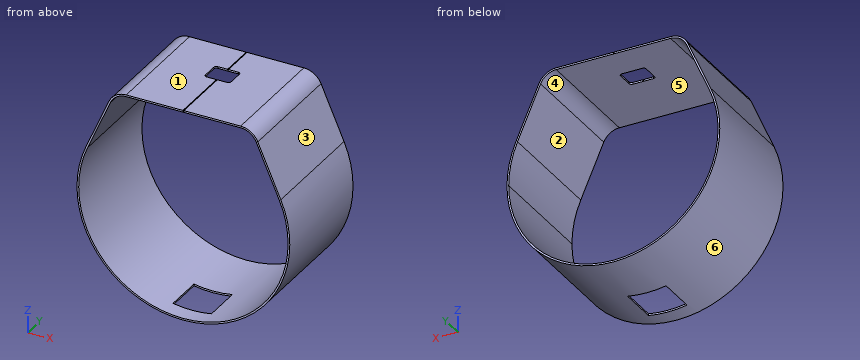
```python
from build123d import *

# Parameters (mm, degrees)
BOSS_EXTRUDE1_DEPTH = 90
CUT_EXTRUDE1_DEPTH  = 22
SKETCH4_W           = 22.5
SKETCH4_H           = 22.5
CUT_EXTRUDE3_DEPTH  = 126.897279558
CUT_EXTRUDE4_DEPTH  = 3
SKETCH6_W           = 0.5
SKETCH6_H           = 68
CUT_EXTRUDE5_DEPTH  = 0.5


# Read off the part's stored shape, not the designer's step: Cut-Extrude1
with BuildPart() as part:
    # Sketch1 → Boss-Extrude1 (new body)
    with BuildSketch(Plane(origin=(0, 0, 0), x_dir=(1, 0, 0), z_dir=(0, 1, 0))):
        with BuildLine():
            ThreePointArc((33.469387755, -62.25), (39.484065665, -60.45997555), (43.541212573, -55.672481752))
            Line((43.541212573, -55.672481752), (56.997372263, -25.027226277))
            ThreePointArc((56.997372263, -25.027226277), (0, 62.25), (-56.997372263, -25.027226277))
            Line((-56.997372263, -25.027226277), (-43.541212573, -55.672481752))
            ThreePointArc((-43.541212573, -55.672481752), (-39.484065665, -60.45997555), (-33.469387755, -62.25))
            Line((-33.469387755, -62.25), (33.469387755, -62.25))
        make_face()
        with BuildLine():
            Line((-9.5e-08, -61.25), (-33.469387755, -61.25))
            ThreePointArc((-33.469387755, -61.25), (-38.937276764, -59.622705046), (-42.625592135, -55.270437956))
            Line((-42.625592135, -55.270437956), (-56.081751825, -24.625182482))
            ThreePointArc((-56.081751825, -24.625182482), (-12.580842594, 59.944014711), (61.25, 0))
            ThreePointArc((61.25, 0), (59.944014711, -12.580842594), (56.081751825, -24.625182482))
            Line((56.081751825, -24.625182482), (42.625592135, -55.270437956))
            ThreePointArc((42.625592135, -55.270437956), (38.937276764, -59.622705046), (33.469387755, -61.25))
            Line((33.469387755, -61.25), (-9.5e-08, -61.25))
        make_face(mode=Mode.SUBTRACT)
    extrude(amount=BOSS_EXTRUDE1_DEPTH)

    # Cut-Extrude1 outline → Cut-Extrude1 (cut)
    with BuildSketch(Plane(origin=(0, 0, 0), x_dir=(1, 0, 0), z_dir=(0, 1, 0))):
        with BuildLine():
            Line((43.541212573, -55.672481752), (56.997372263, -25.027226277))
            ThreePointArc((56.997372263, -25.027226277), (0, 62.25), (-56.997372263, -25.027226277))
            Line((-56.997372263, -25.027226277), (-43.541212573, -55.672481752))
            ThreePointArc((-43.541212573, -55.672481752), (-39.484065665, -60.45997555), (-33.469387755, -62.25))
            Line((-33.469387755, -62.25), (33.469387755, -62.25))
            ThreePointArc((33.469387755, -62.25), (39.484065665, -60.45997555), (43.541212573, -55.672481752))
        make_face()
        with BuildLine():
            Line((33.469387755, -61.25), (-33.469387755, -61.25))
            ThreePointArc((-33.469387755, -61.25), (-38.937276765, -59.622705046), (-42.625592135, -55.270437956))
            Line((-42.625592135, -55.270437956), (-56.081751825, -24.625182482))
            ThreePointArc((-56.081751825, -24.625182482), (0, 61.25), (56.081751825, -24.625182482))
            Line((56.081751825, -24.625182482), (42.625592135, -55.270437956))
            ThreePointArc((42.625592135, -55.270437956), (38.937276765, -59.622705046), (33.469387755, -61.25))
        make_face(mode=Mode.SUBTRACT)
    extrude(amount=CUT_EXTRUDE1_DEPTH, mode=Mode.SUBTRACT)

    # Sketch4 → Cut-Extrude3 (cut, through all)
    with BuildSketch(Plane.XY):
        with Locations((0, 42.75)):
            Rectangle(SKETCH4_W, SKETCH4_H)
    extrude(amount=-CUT_EXTRUDE3_DEPTH, mode=Mode.SUBTRACT)

    # Sketch5 → Cut-Extrude4 (cut)
    with BuildSketch(Plane.XY.offset(62.25)):
        with BuildLine():
            Line((-6, 58), (6, 58))
            ThreePointArc((6, 58), (7.060660172, 58.439339828), (7.5, 59.5))
            Line((7.5, 59.5), (7.5, 68.5))
            ThreePointArc((7.5, 68.5), (7.060660172, 69.560660172), (6, 70))
            Line((6, 70), (-6, 70))
            ThreePointArc((-6, 70), (-7.060660172, 69.560660172), (-7.5, 68.5))
            Line((-7.5, 68.5), (-7.5, 59.5))
            ThreePointArc((-7.5, 59.5), (-7.060660172, 58.439339828), (-6, 58))
        make_face()
    extrude(amount=-CUT_EXTRUDE4_DEPTH, mode=Mode.SUBTRACT)

    # Sketch6 → Cut-Extrude5 (cut)
    with BuildSketch(Plane.XY.offset(62.25)):
        with Locations((0, 56)):
            Rectangle(SKETCH6_W, SKETCH6_H)
    extrude(amount=-CUT_EXTRUDE5_DEPTH, mode=Mode.SUBTRACT)


solid = part.part
```
Geometry check sheet. Reference: the model listing, model coordinates, mm. Face numbers are marked on the shaded views. A direction names the side the tool comes from. Give positions to 0.01 mm unless a question says otherwise; leave off trailing zeros. Write each loop counter-clockwise with the first axis right and the second up, starting at its lowest first coordinate (ties: lowest second). Pieces come first, ordered by that corner, then holes. Notation, with made-up numbers: (-19.5, 39.25) -> (27.5, 39.25) arc R28 cw to (27.5, 77.25) -> close; hole circle Ø3 at (-32.75, 41). An arc over 180 degrees is marked (long way). One line per question, with ' | ' between items.
Item 1: Sectioned sample at A-A, the plane y = 83. Record the boundary of the cut face in (x, z), plus the area to 3 significant figures.
Determined:
outline: (-57, 25.03) arc R62.25 ccw (long way) to (57, 25.03) -> (43.54, 55.67) arc R11 ccw to (33.47, 62.25) -> (0.25, 62.25) -> (0.25, 61.75) -> (-0.25, 61.75) -> (-0.25, 62.25) -> (-33.47, 62.25) arc R11 ccw to (-43.54, 55.67) -> close; hole (-56.08, 24.63) arc R61.25 ccw (long way) to (56.08, 24.63) -> (42.63, 55.27) arc R10 ccw to (33.47, 61.25) -> (-33.47, 61.25) arc R10 ccw to (-42.63, 55.27) -> close | area: 403 mm^2
Item 2: Sectioned sample at B-B, the plane x = -16. Record the boundary of the cut face in (y, z), plus the area to 3 significant figures.
Determined:
outline: (22, -60.16) -> (90, -60.16) -> (90, -59.12) -> (22, -59.12) -> close; (22, 61.25) -> (90, 61.25) -> (90, 62.25) -> (22, 62.25) -> close | area: 138 mm^2
Item 3: Access from +Z, -Z, +X, -X, +Y, -Y to the whole of each face (thin tool, end or side, straight path). Record for the marked faces 1 and 2.
Determined:
face 1: +Z, +X, -X, +Y, -Y | face 2: +Y, -Y
Item 4: Depth check by flat-ended pin: pin 1 (1.5 mm diameter, centred on y = 74.5, z = 48, fed in from +X); pin 2 (1.5 mm diameter, centred on x = 33.5, y = 67.5, fed in from -Z); pin 3 (0.5 mm diameter, centred on y = 65.5, z = 61.5, fed in from +X); pin 4 (2 mm diameter, centred on x = -0.5, z = -61, fed in from -Y). Enter the tip coordinate at first touch or a pass-through.
Determined:
pin 1: x = 47.24 | pin 2: z = -52.94 | pin 3: x = 38.05 | pin 4: y = 22
Item 5: Scan lines: line 1 along X through (y, z) = (54.5, 0); line 2 along Z through (x, y) = (0, 57.5); line 3 along Z through (x, y) = (0.5, 48.5). Record each from-to range of solid material in increasing order.
Determined:
line 1: -62.25 to -61.25, 61.25 to 62.25 | line 2: -62.25 to -61.25, 61.25 to 61.75 | line 3: 61.25 to 62.25
Item 6: Draft check along Z on the marked faces 3, 4, 5 and 6. Enter one of: released by +Z, released by -Z, zero draft, split by the parting line, or undercut.
Determined:
face 3: released by +Z | face 4: undercut | face 5: undercut | face 6: split by the parting line
Item 7: Sectioned sample at D-D, the plane y = 65. Record the boundary of the cut face in (x, z).
Determined:
outline: (-57, 25.03) arc R62.25 ccw (long way) to (57, 25.03) -> (43.54, 55.67) arc R11 ccw to (33.47, 62.25) -> (7.5, 62.25) -> (7.5, 61.25) -> (33.47, 61.25) arc R10 cw to (42.63, 55.27) -> (56.08, 24.63) arc R61.25 cw (long way) to (-56.08, 24.63) -> (-42.63, 55.27) arc R10 cw to (-33.47, 61.25) -> (-7.5, 61.25) -> (-7.5, 62.25) -> (-33.47, 62.25) arc R11 ccw to (-43.54, 55.67) -> close
Item 8: Sectioned sample at C-C, the plane z = 30.5. Record the boundary of the cut face in (x, y).
Determined:
outline: (-54.59, 22) -> (-53.5, 22) -> (-53.5, 90) -> (-54.59, 90) -> close; (53.5, 22) -> (54.59, 22) -> (54.59, 90) -> (53.5, 90) -> close
